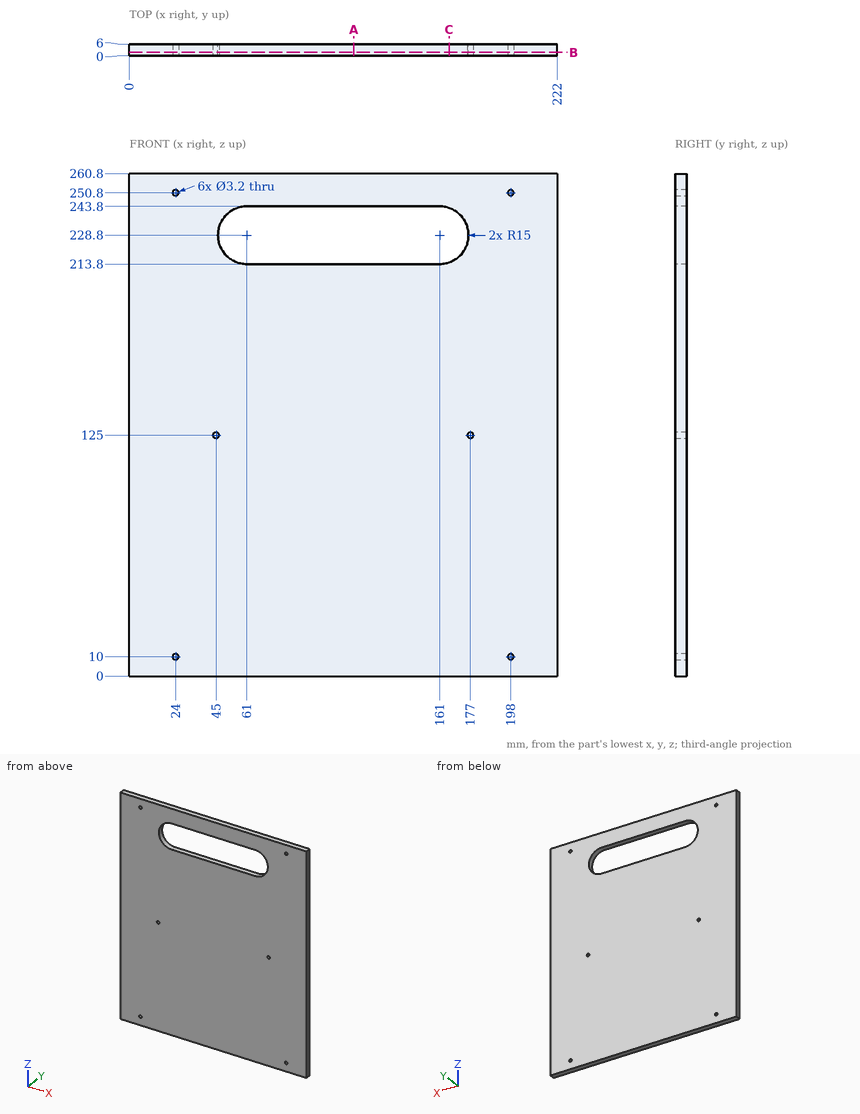
The drawing under review shows one solid part. Ordinate dimensions are in mm from its lowest x, y, z. Round coordinates to 2 decimals unless told otherwise and drop trailing zeros. Order: outer loops, then holes, each group sorted by start corner. A loop starts at its lowest first (then second) coordinate and runs counter-clockwise, first axis right, second up. Notation, with made-up numbers: (82, 71) -> (108, 71) arc R15 cw to (108, 87) -> close; hole circle Ø10 at (53, 4). An arc over 180 degrees is marked (long way). Use a Markdown table: item, result.
Item 1: For pin 1 (1.9 mm diameter, centred on x = 45, z = 125, fed in from -Y), flat-tipped, find the tip position at first contact; note if it passes through.
Resolved:
| item | result |
|---|---|
| pin 1 | passes through |
Item 2: Take a section at A-A (x = 116.5). State the section outline as (y, z) points.
Resolved:
| item | result |
|---|---|
| outline | (0, 0) -> (6, 0) -> (6, 213.8) -> (0, 213.8) -> close; (0, 243.8) -> (6, 243.8) -> (6, 260.8) -> (0, 260.8) -> close |
Item 3: Take a section at C-C (x = 166). State the section outline as (y, z) points, plus the area to 3 significant figures.
Resolved:
| item | result |
|---|---|
| outline | (0, 0) -> (6, 0) -> (6, 214.66) -> (0, 214.66) -> close; (0, 242.94) -> (6, 242.94) -> (6, 260.8) -> (0, 260.8) -> close |
| area | 1,400 mm² |
Item 4: Take a section at B-B (y = 1.65). State the section outline as (x, z) points.
Resolved:
| item | result |
|---|---|
| outline | (0, 0) -> (222, 0) -> (222, 260.8) -> (0, 260.8) -> close; hole circle Ø3.2 at (24, 10); hole circle Ø3.2 at (24, 250.8); hole circle Ø3.2 at (45, 125); hole (61, 213.8) -> (161, 213.8) arc R15 ccw to (161, 243.8) -> (61, 243.8) arc R15 ccw to start; hole circle Ø3.2 at (177, 125); hole circle Ø3.2 at (198, 10); hole circle Ø3.2 at (198, 250.8) |
Item 5: For line 1 along X through (y, z) = (3.1, 125); line 2 along Z through (x, y) = (177, 4.15); line 3 along Z through (x, y) = (134.5, 3.95), list the stretches that pass through material, from the lowest coordinate up. Write a range as [from, to].
Resolved:
| item | result |
|---|---|
| line 1 | x = [0, 43.4], [46.6, 175.4], [178.6, 222] |
| line 2 | z = [0, 123.4], [126.6, 260.8] |
| line 3 | z = [0, 213.8], [243.8, 260.8] |
